Geometry: final body of the model. Coordinates: model frame, mm. Coordinates: 2 decimals unless noted, no trailing zeros. Write each loop counter-clockwise with the first axis right and the second up, starting at its lowest first coordinate (ties: lowest second). Pieces come first, ordered by that corner, then holes. Notation, with made-up numbers: (57.25, -11) - (70.25, -11) arc R35 cw to (70.25, 26) - close; hole circle Ø5 at (5.25, -5). An arc over 180 degrees is marked (long way). Put each result on its own line as item: value.
```python
from build123d import *

# Parameters (mm, degrees)
SKETCH7_W                   = 30
SKETCH7_H                   = 30
THICKEN5_T2                 = 1
BODY_MOVE_COPY5_START       = 35.102954004
BODY_MOVE_COPY5_OUTLINE_W   = 30
BODY_MOVE_COPY5_OUTLINE_H   = 30
BODY_MOVE_COPY5_DEPTH       = 0.011205152
BODY_MOVE_COPY5_START_2     = 34.102954004
BODY_MOVE_COPY5_2_OUTLINE_W = 30
BODY_MOVE_COPY5_2_OUTLINE_H = 30
BODY_MOVE_COPY5_2_DEPTH     = 0.011205152


# Read off the part's stored shape, not the designer's step: Thicken1, Body-Move/Copy5
with BuildPart() as part:
    # Thicken1 outline → Thicken1 (revolve)
    with BuildSketch(Plane(origin=(-5.431630681, 0, 0), x_dir=(1, 0, 0), z_dir=(0, 0, 1))):
        Polygon((4.120349674, 1.929400611), (4.136521177, -0.904564978), (4.936508153, -0.9), (4.918558927, 2.245501685), (3.3, 3.988409531), (3.3, 4.088409531), (5, 5.913409531), (3.3, 7.738409531), (3.3, 7.838409531), (5, 9.663409531), (3.3, 11.488409531), (3.3, 11.588409531), (5, 13.413409531), (3.3, 15.238409531), (3.3, 15.338409531), (5, 17.163409531), (3.3, 18.988409531), (3.3, 19.088409531), (5, 20.913409531), (3.3, 22.738409531), (3.3, 22.838409531), (5, 24.663409531), (3.3, 26.488409531), (3.3, 26.588409531), (5, 28.413409531), (3.3, 30.238409531), (3.3, 30.338409531), (5, 32.163409531), (3.3, 33.988409531), (3.3, 34.102954004), (0, 34.102954004), (0, 33.302954004), (2.845194483, 33.302954004), (3.906687965, 32.163409531), (2.5, 30.653288628), (2.5, 29.923530434), (3.906687965, 28.413409531), (2.5, 26.903288628), (2.5, 26.173530434), (3.906687965, 24.663409531), (2.5, 23.153288628), (2.5, 22.423530434), (3.906687965, 20.913409531), (2.5, 19.403288628), (2.5, 18.673530434), (3.906687965, 17.163409531), (2.5, 15.653288628), (2.5, 14.923530434), (3.906687965, 13.413409531), (2.5, 11.903288628), (2.5, 11.173530434), (3.906687965, 9.663409531), (2.5, 8.153288628), (2.5, 7.423530434), (3.906687965, 5.913409531), (2.5, 4.403288628), (2.5, 3.674236782), align=None)
    revolve(axis=Axis((-5.431630681, 0, 0), (0, 1, 0)))


with BuildPart() as body_2:
    # Sketch7 → Surface-Plane3: a flat surface bounded by the sketch
    with BuildSketch(Plane(origin=(0, 0, 0), x_dir=(1, 0, 0), z_dir=(0, 1, 0)), mode=Mode.PRIVATE) as surface_plane3_1_region:
        with Locations((44.749783052, 15)):
            Rectangle(SKETCH7_W, SKETCH7_H)
    surface_plane3_1 = surface_plane3_1_region.sketch.faces()[0]
    add(Solid.thicken(surface_plane3_1, -THICKEN5_T2))


with BuildPart() as body_2_1:
    # Body-Move/Copy3: moved
    add(body_2.part.moved(Location((-50.300030874, 35.114159156, 14.96319027))))

    # Body-Move/Copy5 outline → Body-Move/Copy5 (cut)
    with BuildSketch(Plane(origin=(0, 0, 0), x_dir=(1, 0, 0), z_dir=(0, 1, 0)).offset(BODY_MOVE_COPY5_START)):
        with Locations((-5.550247822, 0.03680973)):
            Rectangle(BODY_MOVE_COPY5_OUTLINE_W, BODY_MOVE_COPY5_OUTLINE_H)
    extrude(amount=BODY_MOVE_COPY5_DEPTH, mode=Mode.SUBTRACT)

    # Body-Move_Copy5 2 outline → Body-Move_Copy5 2 (add)
    with BuildSketch(Plane(origin=(0, 0, 0), x_dir=(1, 0, 0), z_dir=(0, 1, 0)).offset(BODY_MOVE_COPY5_START_2)):
        with Locations((-5.550247822, 0.03680973)):
            Rectangle(BODY_MOVE_COPY5_2_OUTLINE_W, BODY_MOVE_COPY5_2_OUTLINE_H)
    extrude(amount=BODY_MOVE_COPY5_2_DEPTH)

    # Combine1: union part
    add(part.part)


solid = body_2_1.part
```
1. Pin query (flat end, axial travel): pin 1 Ø1.5 at (x, z) = (4.5, 3) entering from -Y; pin 2 Ø3 at (x, z) = (-5.43, 0) entering from -Y; pin 3 Ø2 at (x, y) = (-6.5, 19) entering from +Z. Return the tip coordinate at first contact, or that it passes through.
Answer below:
pin 1: stops at y = 34.1
pin 2: stops at y = 33.3
pin 3: stops at z = 4.11
2. Section query B-B (y = 27.5). Return loops of the section in (x, z), then the cut area to 3 significant figures.
Answer below:
outline: circle Ø8.3 at (-5.43, 0); hole circle Ø6.11 at (-5.43, 0)
area: 24.7 mm²
3. Section query A-A (x = 3). Return loops of the section in (y, z), then the cut area to 3 significant figures.
Answer below:
outline: (34.1, -15.04) - (35.1, -15.04) - (35.1, 14.96) - (34.1, 14.96) - close
area: 30.0 mm²
4. Mould query, pull axis Z, two halves, no side actions, for faces 1 (the conical face through (-6.17, 26.703, 3.325)), 2 (the cylindrical face through (-3.047, 4.034, -0.751)), 3 (the flat face through (-6, 35.103, 0)). Classes: +Z half, -Z half, draft (parallel to the pull), parting line (faces both ways), or undercut.
Answer below:
face 1: parting line
face 2: undercut
face 3: draft
5. Ray query, probe 1 along Y at (x, z) = (-8, -12.25); probe 2 along Z at (x, y) = (-2.5, 31.5); probe 3 along Z at (x, y) = (-7, 26.5). Return the intervals inside material, ascending. Write a range as from..to.
Answer below:
probe 1: y = 34.1..35.1
probe 2: z = -3.26..-1.49, 1.49..3.26
probe 3: z = -2.9..-1.95, 1.95..2.9
6. Section query C-C (z = -11.25). Return loops of the section in (x, y), then the cut area to 3 significant figures.
Answer below:
outline: (-20.55, 34.1) - (9.45, 34.1) - (9.45, 35.1) - (-20.55, 35.1) - close
area: 30.0 mm²
7. Section query D-D (y = 31.5). Return loops of the section in (x, z), then the cut area to 3 significant figures.
Answer below:
outline: circle Ø8.76 at (-5.43, 0); hole circle Ø6.58 at (-5.43, 0)
area: 26.3 mm²
